The figure shows three views and two pictorial views of one solid part (mm, origin at its lowest corner). Answer the questions. A direction names the side the tool comes from. Coordinates: 2 decimals unless noted, no trailing zeros. Write each loop counter-clockwise with the first axis right and the second up, starting at its lowest first coordinate (ties: lowest second). Pieces come first, ordered by that corner, then holes.
Item 1: This flat-tipped pin is pushed along its axis until it touches: P1, Ø1, axis at x = 8.5, y = 10.5, coming from the -Z side. Where does it stop, or does it pass through?
Item 2: A tool of negligible diameter and unlimited length cuts with its end or side. For the marked faces 4 and 5, from which of +Z, -Z, +X, -X, +Y, -Y can it reach the whole face along a straight path? Write none if from no direction.
Item 3: Section A-A (z = 0.3) is taken. Give the vertices of the cut face in (x, y).
Item 4: Section B-B (y = 3) is taken. Give the vertices of the cut face in (x, z).
Item 5: Straight lines are drawn through the part: probe 1 along Y at (x, z) = (0.5, 0.2); probe 2 along Y at (x, z) = (9, 0.2); probe 3 along Y at (x, z) = (1.75, 0.3). For each, find the intervals that lie inside material, in ascending order.
Item 6: Determine the mould class of the marked faces 1, 2 and 3 for opening direction Y: released by +Y, released by -Y, zero draft, split by the parting line, or undercut.
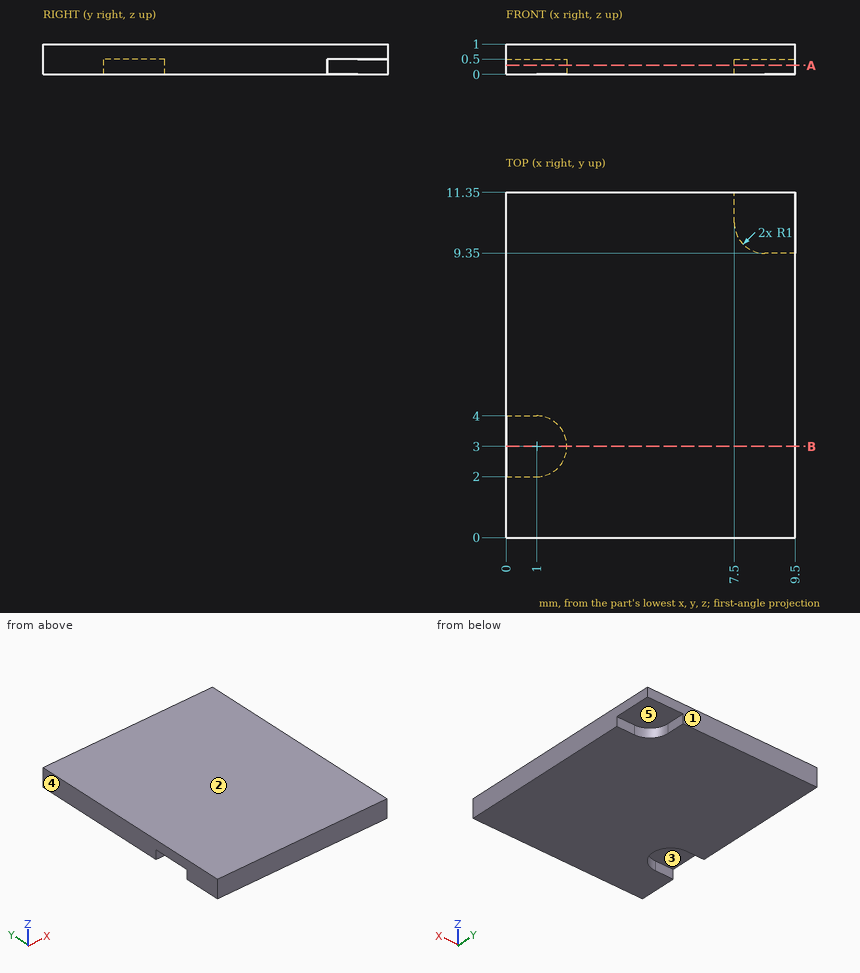
Established:
1. P1: stops at z = 0.5
2. face 4: +Z, -Z, -X, +Y, -Y
2. face 5: -Z, +X, +Y
3. outline: (0, 0) - (9.5, 0) - (9.5, 9.35) - (8.5, 9.35) arc R1 cw to (7.5, 10.35) - (7.5, 11.35) - (0, 11.35) - (0, 4) - (1, 4) arc R1 cw to (1, 2) - (0, 2) - close
4. outline: (0, 0.5) - (2, 0.5) - (2, 0) - (9.5, 0) - (9.5, 1) - (0, 1) - close
5. probe 1: y = 0 to 2, 4 to 11.35
5. probe 2: y = 0 to 9.35
5. probe 3: y = 0 to 2.34, 3.66 to 11.35
6. face 1: released by +Y
6. face 2: zero draft
6. face 3: undercut
